Work out the finished part from the listing and answer in its coordinate system (mm). A direction names the side the tool comes from. Coordinates: 2 decimals unless noted, no trailing zeros. Loops run counter-clockwise (first coordinate to the right, second up) from the corner with the lowest first, then second, coordinate; pieces in that order, holes last. Notation, with made-up numbers: (46, 46.25) -> (85, 46.25) arc R25 cw to (85, 59.25) -> close; hole circle Ø1 at (63, -27). An arc over 180 degrees is marked (long way). One line per question, with ' | ' between items.
```python
from build123d import *

# Parameters (mm, degrees)
SHELL1_T = -5


with BuildPart() as part:
    # Sketch1 → Revolve1 (revolve)
    with BuildSketch(Plane(origin=(0, 0, 0), x_dir=(0, 0, -1), z_dir=(1, 0, 0))):
        Polygon((0, 329.971145898), (0, -70.028854102), (-150, -70.028854102), (-150, 319.971145898), (-190, 319.971145898), (-190, 329.971145898), align=None)
    revolve(axis=Axis((0, 438.369922809, 0), (0, -1, 0)))

    # Shell1
    shell1_openings = [part.faces().sort_by_distance(p)[0] for p in [
        (0, 329.971145898, 0),
    ]]
    offset(amount=SHELL1_T, openings=shell1_openings, kind=Kind.INTERSECTION)


solid = part.part
```
1) Flat-ended cylindrical pins translate along their axes: pin 1 (10 mm diameter, centred on x = 112.5, z = 103.5, fed in from -Y); pin 2 (1.5 mm diameter, centred on x = 42, y = 60, fed in from -Z); pin 3 (6 mm diameter, centred on x = 65, y = 213.5, fed in from +Z); pin 4 (8 mm diameter, centred on x = 72, y = 6, fed in from -Z). Find the tip coordinate at first contact, or state that the pin passes through.
Check values:
pin 1: stops at y = -70.03 | pin 2: stops at z = -144.22 | pin 3: stops at z = 136.59 | pin 4: stops at z = -133.7
2) Find section A-A (z = 0). Write down the section's boundary in (x, y).
Check values:
outline: (-190, 319.97) -> (-150, 319.97) -> (-150, -70.03) -> (150, -70.03) -> (150, 319.97) -> (190, 319.97) -> (190, 329.97) -> (185, 329.97) -> (185, 324.97) -> (145, 324.97) -> (145, -65.03) -> (-145, -65.03) -> (-145, 324.97) -> (-185, 324.97) -> (-185, 329.97) -> (-190, 329.97) -> close
3) For faces 1 (the face through (182, 329.971, 41)), 2 (the face through (-155.993, 327.506, 99.455)), 3 (the face through (-57, 319.971, -140)), determine the directions among +Z, -Z, +X, -X, +Y, -Y from which every point of the face is accessible in a straight line to the end or side of a thin tool.
Check values:
face 1: +Z, -Z, +X, -X, +Y | face 2: +Y | face 3: -Y
4) Find section B-B (y = -33.5). Write down the section's boundary in (x, z), plus the area to 3 significant figures.
Check values:
outline: circle Ø300 at (0, 0); hole circle Ø290 at (0, 0) | area: 4,630 mm^2
5) Find section D-D (z = 157). Write down the section's boundary in (x, y).
Check values:
outline: (-107.01, 319.97) -> (107.01, 319.97) -> (107.01, 329.97) -> (97.86, 329.97) -> (97.86, 324.97) -> (-97.86, 324.97) -> (-97.86, 329.97) -> (-107.01, 329.97) -> close
6) Find the intervals of material crossed by line 1 along X through (y, z) = (104, 0); line 2 along X through (y, z) = (327.35, 0); line 3 along Y through (x, z) = (73.5, 18), in increasing order.
Check values:
line 1: x = -150 to -145, 145 to 150 | line 2: x = -190 to -185, 185 to 190 | line 3: y = -70.03 to -65.03
7) Find section C-C (x = 0). Write down the section's boundary in (y, z).
Check values:
outline: (-70.03, -150) -> (319.97, -150) -> (319.97, -190) -> (329.97, -190) -> (329.97, -185) -> (324.97, -185) -> (324.97, -145) -> (-65.03, -145) -> (-65.03, 145) -> (324.97, 145) -> (324.97, 185) -> (329.97, 185) -> (329.97, 190) -> (319.97, 190) -> (319.97, 150) -> (-70.03, 150) -> close
8) The mould has two halves that part along X. Classify faces 4 (the face through (-2, -70.029, 2)), 5 (the face through (185.48, 325.04, -41.19)), 6 (the face through (-2, -65.029, 2)): released by +X, released by -X, zero draft, split by the parting line, or undercut.
Check values:
face 4: zero draft | face 5: split by the parting line | face 6: undercut
